from build123d import *

# Parameters (mm, degrees)
BOSS_EXTRUDE1_DEPTH = 3
FILLET1_R           = 10
SKETCH2_W           = 2.9
SKETCH2_H           = 10
CUT_EXTRUDE1_DEPTH  = 168.247780254


with BuildPart() as part:
    # Sketch1 → Boss-Extrude1 (new body)
    with BuildSketch(Plane.XY):
        Polygon((-69, 54.9), (-69, 0), (-55, 0), (-55, 6), (-45, 6), (-45, 0), (-35, 0), (-35, 6), (-25, 6), (-25, 0), (-15, 0), (-15, 6), (-5, 6), (-5, 0), (5, 0), (5, 6), (15, 6), (15, 0), (25, 0), (25, 6), (35, 6), (35, 0), (45, 0), (45, 6), (55, 6), (55, 0), (69, 0), (69, 54.9), (134.1, 54.9), (134.1, 59.9), (131, 59.9), (131, 69.9), (134.1, 69.9), (134.1, 79.9), (131, 79.9), (131, 89.9), (134.1, 89.9), (134.1, 99.9), (-134.1, 99.9), (-134.1, 89.9), (-131, 89.9), (-131, 79.9), (-134.1, 79.9), (-134.1, 69.9), (-131, 69.9), (-131, 59.9), (-134.1, 59.9), (-134.1, 54.9), align=None)
    extrude(amount=BOSS_EXTRUDE1_DEPTH)

    # Fillet1
    fillet1_edges = [part.edges().sort_by_distance(p)[0] for p in [
        (69, 54.9, 1.5),
        (-69, 54.9, 1.5),
    ]]
    fillet(fillet1_edges, radius=FILLET1_R)

    # Sketch2 → Cut-Extrude1 (cut, through all)
    with BuildSketch(Plane(origin=(0, 0, 0), x_dir=(-1, 0, 0), z_dir=(0, 0, -1))):
        with Locations((-63.702453972, 15)):
            Rectangle(SKETCH2_W, SKETCH2_H)
        with Locations((-63.702453972, 35)):
            Rectangle(SKETCH2_W, SKETCH2_H)
        with Locations((63.702453972, 35)):
            Rectangle(SKETCH2_W, SKETCH2_H)
        with Locations((63.702453972, 15)):
            Rectangle(SKETCH2_W, SKETCH2_H)
    extrude(amount=-CUT_EXTRUDE1_DEPTH, mode=Mode.SUBTRACT)


solid = part.part
Can you work these out from the model? Positions are in its coordinate system, mm. Give positions to 0.01 mm unless a question says otherwise; leave off trailing zeros. Loops run counter-clockwise (first coordinate to the right, second up) from the corner with the lowest first, then second, coordinate; pieces in that order, holes last. Notation, with made-up numbers: (-19, 51) - (-5, 51) arc R28 cw to (-5, 84) - close; hole circle Ø3 at (-8.75, -1). An arc over 180 degrees is marked (long way). Return JSON: item names as keys, results as strings.
1. I want a section at C-C on z = 2.2. Give the number of separate pieces and of enclosed holes in the cut face, and give its area (3 significant figures).
Output values:
{"separate pieces": "1", "enclosed holes": "4", "area": "19,100 mm²"}
2. I want a section at D-D on y = 66.5. Please give me the cut outline in (x, z).
Output values:
{"outline": "(-131, 0) - (131, 0) - (131, 3) - (-131, 3) - close"}
3. I want a section at A-A on y = 16. Please give me the cut outline in (x, z), and give its area (3 significant figures).
Output values:
{"outline": "(-69, 0) - (-65.15, 0) - (-65.15, 3) - (-69, 3) - close; (-62.25, 0) - (62.25, 0) - (62.25, 3) - (-62.25, 3) - close; (65.15, 0) - (69, 0) - (69, 3) - (65.15, 3) - close", "area": "397 mm²"}
4. I want a section at B-B on x = -104. Please give me the cut outline in (y, z).
Output values:
{"outline": "(54.9, 0) - (99.9, 0) - (99.9, 3) - (54.9, 3) - close"}
5. I'm going to push flat-ended pins straight in: pin 1 Ø1.5 at (y, z) = (34, 2) entering from -X; pin 2 Ø0.9 at (x, z) = (-133, 1) entering from -Y; pin 3 Ø1.5 at (y, z) = (64.5, 1) entering from +X. Where does each tip first touch, or does it pass through?
Output values:
{"pin 1": "stops at x = -69", "pin 2": "stops at y = 54.9", "pin 3": "stops at x = 131"}
6. If I drill on line 1 (X direction, y = 19, z = 1.4); line 2 (Y direction, x = -32.5, z = 1.55); line 3 (Y direction, x = -111, z = 2.75), over which ranges is the centre line in solid material (lowest first)?
Output values:
{"line 1": "x = -69 to -65.15, -62.25 to 62.25, 65.15 to 69", "line 2": "y = 6 to 99.9", "line 3": "y = 54.9 to 99.9"}
